Read the model definition and answer for the solid it produces. Units are mm, in the model's axes. Face numbers are marked on the shaded views. A direction names the side the tool comes from. Give positions to 0.01 mm unless a question says otherwise; leave off trailing zeros. Loops run counter-clockwise (first coordinate to the right, second up) from the corner with the lowest first, then second, coordinate; pieces in that order, holes last. Notation, with made-up numbers: (13, 67) - (29, 67) arc R16 ccw to (29, 98) - close; hole circle Ø3 at (60.25, -10.5). An arc over 180 degrees is marked (long way). Use a Markdown table: item, result. Add a question column.
Item 1: A cutting plane is placed at B-B (y = 7.5). Determine the outline of the cut face in (x, z).
Item 2: A cutting plane is placed at D-D (y = -0.5). Determine the outline of the cut face in (x, z), plus the area to 3 significant figures.
Item 3: Consider probe 1 along Y at (x, z) = (-0.25, 3.25); probe 2 along Z at (x, y) = (3.5, -0.5); probe 3 along Y at (x, z) = (-1, 6.75). Determine where each line is inside the solid, lowest interval first. Write a range as [from, to].
Item 4: Which of the six approach directions +Z, -Z, +X, -X, +Y, -Y give full straight-line access (tool end or side, diameter ignored) to the marked faces 1 and 2?
Item 5: A cutting plane is placed at A-A (x = 0). Determine the outline of the cut face in (y, z).
Item 6: A cutting plane is placed at C-C (z = 1). Determine the outline of the cut face in (x, y), plus the area to 3 significant figures.
Item 7: For a pull along X with two mould halves and no side action, classify the marked faces 3, 4, 5 and 6 as +X half, -X half, draft (parallel to the pull), parting line (faces both ways), or undercut.
Item 8: Each of these flat-tipped pins is pushed along its axis until it touches: P1, Ø10, axis at x = -1, y = -2.5, coming from the -Z side; P2, Ø1, axis at x = 5, z = 3, coming from the +Y side; P3, Ø3, axis at x = -4.5, z = 6.5, coming from the -Y side; P4, Ø1.7, axis at x = 4, y = -3.5, coming from the -Z side. Where does it stop, or does it pass through?
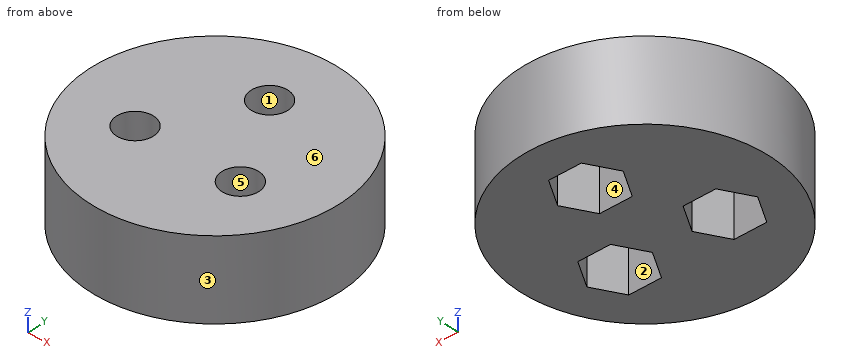
from build123d import *

# Parameters (mm, degrees)
SKETCH1_R           = 12.5
BOSS_EXTRUDE1_DEPTH = 8
SKETCH2_R           = 1.85
CUT_EXTRUDE1_DEPTH  = 8
CUT_EXTRUDE2_DEPTH  = 5
CIRPATTERN1_COUNT   = 3


with BuildPart() as part:
    # Sketch1 → Boss-Extrude1 (new body)
    with BuildSketch(Plane.XY):
        Circle(SKETCH1_R)
    extrude(amount=BOSS_EXTRUDE1_DEPTH)

    # Sketch2 → Cut-Extrude1 (cut)
    with BuildSketch(Plane.XY.offset(8)):
        with Locations((0, 6)):
            Circle(SKETCH2_R)
    cut_extrude1 = extrude(amount=-CUT_EXTRUDE1_DEPTH, mode=Mode.SUBTRACT)

    # Sketch3 → Cut-Extrude2 (cut)
    with BuildSketch(Plane(origin=(0, 0, 0), x_dir=(-1, 0, 0), z_dir=(0, 0, -1))):
        Polygon((3.233161507, 6), (1.616580754, 8.8), (-1.616580754, 8.8), (-3.233161507, 6), (-1.616580754, 3.2), (1.616580754, 3.2), align=None)
    cut_extrude2 = extrude(amount=-CUT_EXTRUDE2_DEPTH, mode=Mode.SUBTRACT)

    # CirPattern1: Cut-Extrude1, Cut-Extrude2 ×3 about axis
    cirpattern1_axis = Axis((0, 0, 0), (0, 0, 1))
    for i in range(1, CIRPATTERN1_COUNT):
        add(cut_extrude1.rotate(cirpattern1_axis, i * 360 / CIRPATTERN1_COUNT), mode=Mode.SUBTRACT)
        add(cut_extrude2.rotate(cirpattern1_axis, i * 360 / CIRPATTERN1_COUNT), mode=Mode.SUBTRACT)


solid = part.part
Geometry says:
| question | item | result |
|---|---|---|
| 1 | outline | (-10, 0) - (-2.37, 0) - (-2.37, 5) - (-1.08, 5) - (-1.08, 8) - (-10, 8) - close; (1.08, 5) - (2.37, 5) - (2.37, 0) - (10, 0) - (10, 8) - (1.08, 8) - close |
| 2 | outline | (-12.49, 0) - (-6.99, 0) - (-6.99, 5) - (-3.41, 5) - (-3.41, 0) - (3.41, 0) - (3.41, 5) - (6.99, 5) - (6.99, 0) - (12.49, 0) - (12.49, 8) - (-12.49, 8) - close |
| 2 | area | 164 mm² |
| 3 | probe 1 | [-12.5, 3.2], [8.8, 12.5] |
| 3 | probe 2 | [5, 8] |
| 3 | probe 3 | [-12.46, 4.44], [7.56, 12.46] |
| 4 | face 1 | +Z, -Z |
| 4 | face 2 | -Z |
| 5 | outline | (-12.5, 0) - (3.2, 0) - (3.2, 5) - (4.15, 5) - (4.15, 8) - (-12.5, 8) - close; (7.85, 5) - (8.8, 5) - (8.8, 0) - (12.5, 0) - (12.5, 8) - (7.85, 8) - close |
| 6 | outline | circle Ø25 at (0, 0); hole (-8.43, -3) - (-6.81, -5.8) - (-3.58, -5.8) - (-1.96, -3) - (-3.58, -0.2) - (-6.81, -0.2) - close; hole (-3.23, 6) - (-1.62, 3.2) - (1.62, 3.2) - (3.23, 6) - (1.62, 8.8) - (-1.62, 8.8) - close; hole (1.96, -3) - (3.58, -5.8) - (6.81, -5.8) - (8.43, -3) - (6.81, -0.2) - (3.58, -0.2) - close |
| 6 | area | 409 mm² |
| 7 | face 3 | parting line |
| 7 | face 4 | undercut |
| 7 | face 5 | undercut |
| 7 | face 6 | draft |
| 8 | P1 | z = 0 |
| 8 | P2 | y = 11.66 |
| 8 | P3 | y = -12.13 |
| 8 | P4 | z = 5 |
